Read the model definition and answer for the solid it produces. Units are mm, in the model's axes. A direction names the side the tool comes from. Coordinates: 2 decimals unless noted, no trailing zeros. Loops run counter-clockwise (first coordinate to the right, second up) from the corner with the lowest first, then second, coordinate; pieces in that order, holes last. Notation, with made-up numbers: (72.5, 20.5) - (88.5, 20.5) arc R7 cw to (88.5, 25.5) - close; hole circle Ø11 at (-27.5, -30). An arc over 180 degrees is marked (long way). Use one line per item in the form item = value. Start each with the question number.
1) Which of the six approach directions +Z, -Z, +X, -X, +Y, -Y give full straight-line access (tool end or side, diameter ignored) to faces 5 (the face through (25.4, -501, 13)), 6 (the face through (13, -501, 23.927))?
2) The mould has two halves that part along X. Classify faces 1 (the face through (0, -501, 13)), 2 (the face through (13, -501, 25.4)), 3 (the face through (1.473, -501, 13)), 4 (the face through (13, -501, 1.473)): released by +X, released by -X, zero draft, split by the parting line, or undercut.
3) A cutting plane is placed at C-C (y = -445). Give the vertices of the cut face in (x, z), and give its area (3 significant figures).
4) A cutting plane is placed at A-A (z = 6). Give the vertices of the cut face in (x, y).
5) A cutting plane is placed at B-B (x = 12.7). Give the vertices of the cut face in (y, z), and give its area (3 significant figures).
6) Consider line 1 (X direction, y = -220.5, z = 10.75); line 2 (Y direction, x = 12.7, z = 24.4). Determine where each line is inside the solid, lowest interval first.
from build123d import *

# Parameters (mm, degrees)
F0_W     = 25.4
F0_H     = 25.4
F0_W_2   = 22.4536
F0_H_2   = 22.4536
F1_DEPTH = 1016
F2_R     = 6.35
F3_DEPTH = 25.401


with BuildPart() as f1:
    # F0 (on Front) → F1 (new body)
    with BuildSketch(Plane.XZ):
        with Locations((12.7, 12.7)):
            Rectangle(F0_W, F0_H)
        with Locations((12.7, 12.7)):
            Rectangle(F0_W_2, F0_H_2, mode=Mode.SUBTRACT)
    extrude(amount=F1_DEPTH)

    # F2 (on face) → F3 (cut, through all)
    with BuildSketch(Plane(origin=(0, 0, 0), x_dir=(1, 0, 0), z_dir=(0, 0, -1))):
        with Locations((12.7, 508)):
            Circle(F2_R)
    extrude(amount=-F3_DEPTH, mode=Mode.SUBTRACT)


solid = f1.part
Found:
q1.face_5 = +Z, -Z, +X, +Y, -Y
q1.face_6 = +Y, -Y
q2.face_1 = released by -X
q2.face_2 = zero draft
q2.face_3 = undercut
q2.face_4 = undercut
q3.outline = (0, 0) - (25.4, 0) - (25.4, 25.4) - (0, 25.4) - close; hole (1.47, 1.47) - (23.93, 1.47) - (23.93, 23.93) - (1.47, 23.93) - close
q3.area = 141 mm^2
q4.outline = (0, -1016) - (1.47, -1016) - (1.47, 0) - (0, 0) - close; (23.93, -1016) - (25.4, -1016) - (25.4, 0) - (23.93, 0) - close
q5.outline = (-1016, 0) - (-514.35, 0) - (-514.35, 1.47) - (-1016, 1.47) - close; (-1016, 23.93) - (-514.35, 23.93) - (-514.35, 25.4) - (-1016, 25.4) - close; (-501.65, 0) - (0, 0) - (0, 1.47) - (-501.65, 1.47) - close; (-501.65, 23.93) - (0, 23.93) - (0, 25.4) - (-501.65, 25.4) - close
q5.area = 2,960 mm^2
q6.line_1 = 0 to 1.47, 23.93 to 25.4
q6.line_2 = -1016 to -514.35, -501.65 to 0
